Autodesk Inventor part; units mm, degrees
ref_plane "Work Plane2" through (0, 104.14, 0) normal (0, 0, -1) x (-1, 0, 0)
ref_plane "YZ Plane" through (0, 0, 0) normal (1, 0, 0) x (0, 1, 0)
ref_plane "XZ Plane" through (0, 0, 0) normal (0, 1, 0) x (-1, 0, 0)
sketch "Sketch1" plane through (0, 0, 0) normal (0, 1, 0) x (-1, 0, 0)
  circle A0 centre (0, 0) radius 4.445
  dimension "d0" = 8.89
extrude "Extrusion1" add sketch "Sketch1" along normal blind 2.54
sketch "Sketch2" plane through (0, 2.54, 0) normal (0, 1, 0) x (1, 0, 0)
  circle A0 centre (0, 0) radius 4.445
  circle A1 centre (0, 0) radius 2.4384
  dimension "d5" = 4.8768
extrude "Extrusion2" add sketch "Sketch2" along normal blind 101.6 contours A1
sketch "Sketch3" plane through (0, 104.14, 0) normal (0, 1, 0) x (1, 0, 0)
  circle A0 centre (0, 0) radius 2.4384
  point P0 (0, 2.4384)
ref_plane "Work Plane2" through (0, 104.14, 0) normal (0, 0, -1) x (-1, 0, 0)
ref_plane "Work Plane1" through (0, 104.14, -2.4384) normal (0, 0, -1) x (-1, 0, 0)
sketch "Sketch4" plane through (0, 104.14, 0) normal (0, 0, -1) x (-1, 0, 0)
  line L0 (3.175, -4.7625) -> (3.175, 0)
  line L1 (3.175, 0) -> (0, 0)
  line L2 (0, 0.1023) -> (0, 1.7624)
  line L3 (0, 0) -> (3.175, -9.525)
  line L4 (3.175, -4.7625) -> (3.175, -9.525)
  point P0 (0, -104.14)
revolve "Revolution1" cut sketch "Sketch4" angle 360 about axis through (0, 104.2423, 0) along (0, 1, 0)
fillet "Fillet1" radius 0.508 1 edges at (4.445, 0, 0)
properties part number "nail" material "Steel, Galvanized"
The listing builds one solid part. Answer for the finished solid, in the listing's coordinates (mm). A direction names the side the tool comes from. Give positions to 0.01 mm unless a question says otherwise; leave off trailing zeros. Order: outer loops, then holes, each group sorted by start corner. A loop starts at its lowest first (then second) coordinate and runs counter-clockwise, first axis right, second up. Notation, with made-up numbers: (-35, 4) -> (20, 4) arc R27 cw to (20, 38) -> close; hole circle Ø2 at (47, -18). An arc over 180 degrees is marked (long way). Answer as a JSON object with one key per item and string values. Group by question number.
Item 1: Consider L1, parallel to Z at x = 0.25, y = 73; L2, parallel to Y at x = -0.5, z = 2.5; L3, parallel to Y at x = -2.25, z = 3.5. Determine where each line is inside the solid, lowest interval first. Write a range as from..to.
Item 2: Flat-ended cylindrical pins translate along their axes: pin 1 (5 mm diameter, centred on x = -0.5, y = 87.5, fed in from +Z); pin 2 (5 mm diameter, centred on y = 84.5, z = -3, fed in from +X); pin 3 (1 mm diameter, centred on y = 62.5, z = 2, fed in from +X). Find the tip coordinate at first contact, or state that the pin passes through.
Item 3: A tool of negligible diameter and unlimited length cuts with its end or side. For faces 1 (the flat face through (0, 0, 0)), 2 (the cylindrical face through (2.326, 49.022, 0.732)), from which of +Z, -Z, +X, -X, +Y, -Y can it reach the whole face along a straight path? Write none if from no direction.
Item 4: The part is cut by section A-A on y = 85.5. Write down the section's boundary in (x, z), and give its area (3 significant figures).
Result set:
{
 "1": {"L1": "-2.43..2.43", "L2": "0..2.54", "L3": "0.05..2.54"},
 "2": {"pin 1": "z = 2.44", "pin 2": "x = 2.39", "pin 3": "x = 1.92"},
 "3": {"face 1": "+Z, -Z, +X, -X, -Y", "face 2": "+Y"},
 "4": {"outline": "circle Ø4.88 at (0, 0)", "area": "18.7 mm²"}
}
